Read the model definition and answer for the solid it produces. Units are mm, in the model's axes. Face numbers are marked on the shaded views. Give positions to 0.01 mm unless a question says otherwise; leave off trailing zeros. Order: outer loops, then holes, each group sorted by start corner. A loop starts at its lowest first (then second) coordinate and runs counter-clockwise, first axis right, second up. Notation, with made-up numbers: (-39, -12) - (-1, -12) arc R16 ccw to (-1, -6) - close; hole circle Ø8 at (53, 24.25). An arc over 180 degrees is marked (long way). Answer as CSV lines item,"result". Start each with the question number.
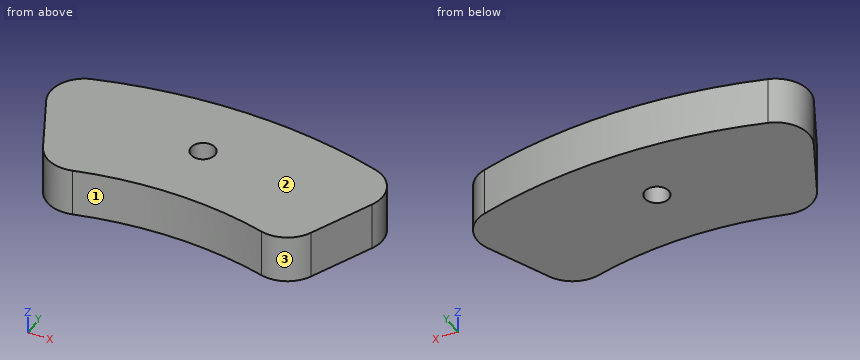
Autodesk Inventor part; units mm, degrees
ref_plane "YZ Plane" through (0, 0, 0) normal (1, 0, 0) x (0, 1, 0)
ref_plane "XZ Plane" through (0, 0, 0) normal (0, 1, 0) x (-1, 0, 0)
ref_plane "XY Plane" through (0, 0, 0) normal (0, 0, 1) x (1, 0, 0)
sketch "Sketch1" plane through (0, 0, 0) normal (0, 0, 1) x (1, 0, 0)
  circle A0 centre (0, 0) radius 45.5
  circle A1 centre (0, 0) radius 52.5
  circle A2 centre (0, 0) radius 38.5
  line L0 (-12.0085, 36.5793) -> (-17.9561, 49.3339)
  line L1 (13.1678, 36.1782) -> (19.101, 48.902)
  line L2 (0, 0) -> (0, 83.0319)
  point P0 (0, 45.5)
  dimension "d2" = 91
  dimension "d3" = 7
  dimension "d4" = 7
  dimension "d5" = 25
  dimension "d6" = 25
extrude "Extrusion1" add sketch "Sketch1" along normal blind 5 contours L1 A2 L2 A0 | A0 L2 A1 L1 | L0 A1 L2 A0 | A0 L2 A2 L0
hole "Hole1" at (0, 45.5, 0) direction (0, 0, 1) diameter 2.5 end through all
fillet "Fillet1" radius 3.5 4 edges at (19.101, 48.902, 2.5) (13.1678, 36.1782, 2.5) (-12.0085, 36.5793, 2.5) (-17.9561, 49.3339, 2.5)
sketch "Sketch2" plane through (0, 0, 5) normal (0, 0, 1) x (1, 0, 0)
  circle A0 centre (0, 0) radius 50
  dimension "d17" = 100
equation "\"d4\" = d3"
equation "\"d6\" = d5"
properties part number "3DP_PLA_Foot"
(1) Determine the mould class of the marked faces 1, 2 and 3 for opening direction X: released by +X, released by -X, zero draft, split by the parting line, or undercut.
(2) Section C-C, the plane y = 41.5 is taken. Write down the section's boundary in (x, z).
(3) Flat-ended cylindrical pins translate along their axes: pin 1 Ø2 at (x, z) = (9, 4.5) entering from -Y; pin 2 Ø1.5 at (x, z) = (12.5, 4) entering from -Y. Find the tip coordinate at first contact, or state that the pin passes through.
(4) Straight lines are drawn through the part: line 1 (Y direction, x = 0, z = 3.95); line 2 (X direction, y = 45.5, z = 1.1); line 3 (X direction, y = 45.25, z = 3.9). For each, find the intervals that lie inside material, in ascending order. Write a range as [from, to].
(5) Section B-B, the plane z = 1.7 is taken. Write down the section's boundary in (x, y), and give its area (3 significant figures).
(6) Section D-D, the plane y = 49.5 is taken. Write down the section's boundary in (x, z), and give its area (3 significant figures).
(7) Section A-A, the plane x = 0 is taken. Write down the section's boundary in (y, z), and give its area (3 significant figures).
Checks:
1,face 1,"undercut"
1,face 2,"zero draft"
1,face 3,"split by the parting line"
2,outline,"(-14.3, 0) - (15.65, 0) - (15.65, 5) - (-14.3, 5) - close"
3,pin 1,"stops at y = 37.18"
3,pin 2,"stops at y = 36.98"
4,line 1,"y = [38.5, 44.25], [46.75, 52.5]"
4,line 2,"x = [-16.17, -1.25], [1.25, 17.51]"
4,line 3,"x = [-16.05, -1.22], [1.22, 17.4]"
5,outline,"(-16.28, 45.74) - (-13.27, 39.29) arc R3.5 ccw to (-9.26, 37.37) arc R38.5 cw to (10.36, 37.08) arc R3.5 ccw to (14.47, 38.97) - (17.46, 45.39) arc R3.5 ccw to (15.31, 50.22) arc R52.5 ccw to (-14.04, 50.59) arc R3.5 ccw to start; hole circle Ø2.5 at (0, 45.5)"
5,area,"429 mm²"
6,outline,"(-15.76, 0) - (16.6, 0) - (16.6, 5) - (-15.76, 5) - close"
6,area,"162 mm²"
7,outline,"(38.5, 0) - (44.25, 0) - (44.25, 5) - (38.5, 5) - close; (46.75, 0) - (52.5, 0) - (52.5, 5) - (46.75, 5) - close"
7,area,"57.5 mm²"
